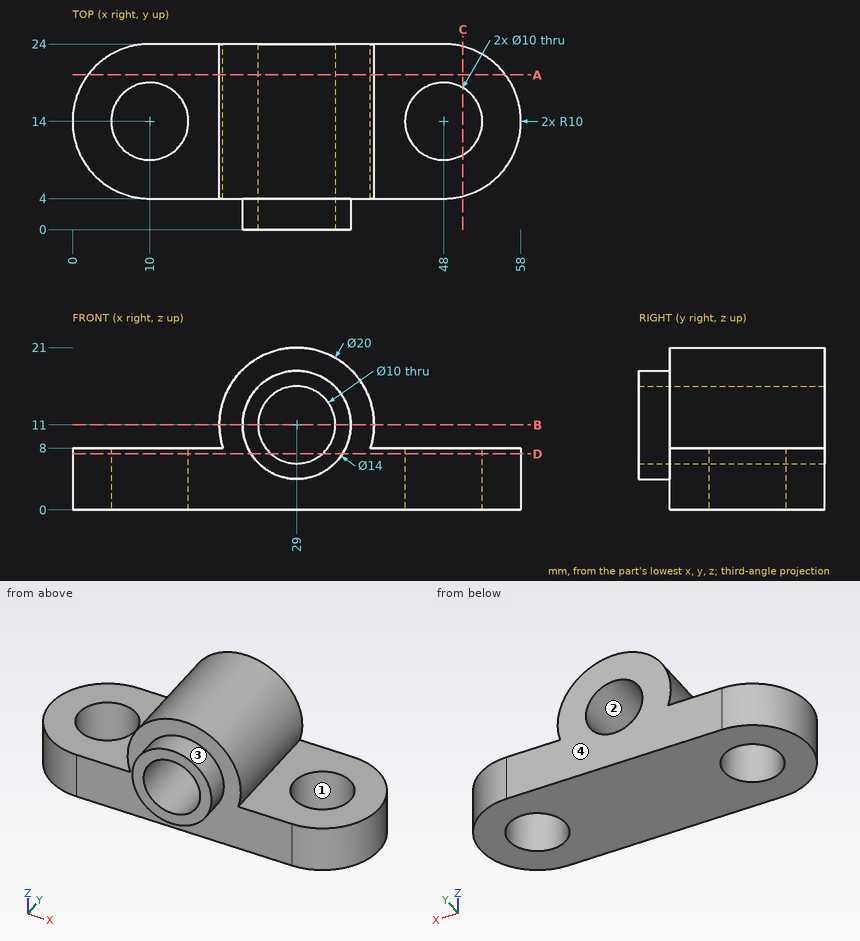
Verification items for this drawing (mm, ordinates from the low corner). Give positions to 0.01 mm unless a question says otherwise; leave off trailing zeros. Loops run counter-clockwise (first coordinate to the right, second up) from the corner with the lowest first, then second, coordinate; pieces in that order, holes last. Notation, with made-up numbers: M 88,-4.75 L 104,-4.75 A23 cw 104,7.25 Z; hole C -31.5,-14 d11. An arc over 180 degrees is marked long. Answer as a JSON object with one key per item and string values. Group by question number.
Q1. Go/stop test with flat-tipped pins: P1, Ø2, axis at x = 22.5, z = 3, coming from the -Y side; P2, Ø6, axis at y = 3.5, z = 8.5, coming from the +X side; P3, Ø1.5, axis at y = 8.5, z = 13.5, coming from the -X side. Record where each tip stops, or that it passes through.
Q2. Cross-section at B-B on z = 11. Record the cut outline in (x, y), then the cut area to 3 significant figures.
Q3. Release check for a two-part mould opening along X. For the marked faces 1, 2, 3 and 4 record: released by +X, released by -X, zero draft, split by the parting line, or undercut.
Q4. Cross-section at D-D on z = 7.25. Record the cut outline in (x, y), then the cut area to 3 significant figures.
Q5. Material ranges on line 1 along Y through (x, z) = (10, 4.5); line 2 along Z through (x, y) = (29, 15.25); line 3 along Z through (x, y) = (50, 7.5), recorded low to high. Write a range as [from, to].
Q6. Cross-section at A-A on y = 20. Record the cut outline in (x, z), then the cut area to 3 significant figures.
Q7. Cross-section at C-C on x = 50.5. Record the cut outline in (y, z), then the cut area to 3 significant figures.
Evaluation:
{
 "1": {"P1": "stops at y = 4", "P2": "stops at x = 54.57", "P3": "stops at x = 19.15"},
 "2": {"outline": "M 19,4 L 22,4 L 22,0 L 24,0 L 24,24 L 19,24 Z; M 34,0 L 36,0 L 36,4 L 39,4 L 39,24 L 34,24 Z", "area": "216 mm2"},
 "3": {"face 1": "undercut", "face 2": "undercut", "face 3": "split by the parting line", "face 4": "zero draft"},
 "4": {"outline": "M 10,4 L 23.09,4 L 23.09,0 L 25.69,0 L 25.69,24 L 10,24 A10 ccw Z; M 32.31,0 L 34.91,0 L 34.91,4 L 48,4 A10 ccw 48,24 L 32.31,24 Z; hole C 10,14 d10; hole C 48,14 d10", "area": "806 mm2"},
 "5": {"line 1": "y = [4, 9], [19, 24]", "line 2": "z = [0, 6], [16, 21]", "line 3": "z = [0, 8]"},
 "6": {"outline": "M 2,0 L 56,0 L 56,8 L 38.54,8 A10 ccw long 19.46,8 L 2,8 Z; hole C 29,11 d10", "area": "570 mm2"},
 "7": {"outline": "M 4.32,0 L 9.67,0 L 9.67,8 L 4.32,8 Z; M 18.33,0 L 23.68,0 L 23.68,8 L 18.33,8 Z", "area": "85.6 mm2"}
}
